```python
from build123d import *

# Parameters (mm, degrees)
BOSS_EXTRUDE1_DEPTH = 10
SKETCH4_R           = 2
CUT_EXTRUDE2_DEPTH  = 10


with BuildPart() as part:
    # Sketch1 → Boss-Extrude1 (new body)
    with BuildSketch(Plane.XY):
        Polygon((33.476154754, 62), (-33.476154754, 62), (-33.5, 62), (-33.5, 3), (-48.5, 3), (-48.5, 0), (-28.5, 0), (-28.5, 57), (28.5, 57), (28.5, 0), (48.5, 0), (48.5, 3), (33.5, 3), (33.5, 62), align=None)
    extrude(amount=BOSS_EXTRUDE1_DEPTH)

    # Sketch4 → Cut-Extrude2 (cut)
    with BuildSketch(Plane(origin=(0, 0, 0), x_dir=(1, 0, 0), z_dir=(0, 1, 0))):
        with Locations((-41.522360656, -5)):
            Circle(SKETCH4_R)
        with Locations((41.522360656, -5)):
            Circle(SKETCH4_R)
    extrude(amount=CUT_EXTRUDE2_DEPTH, mode=Mode.SUBTRACT)


solid = part.part
```
Input: part model. Units: mm. Frame: model coordinates. A direction names the side the tool comes from. Give positions to 0.01 mm unless a question says otherwise; leave off trailing zeros. Loops run counter-clockwise (first coordinate to the right, second up) from the corner with the lowest first, then second, coordinate; pieces in that order, holes last. Notation, with made-up numbers: (58, 44) -> (90, 44) arc R18 ccw to (90, 77) -> close; hole circle Ø7 at (-30, 89). An arc over 180 degrees is marked (long way). Use a Markdown table: item, result.
Q1. Section query B-B, the plane z = 5. Return the cut outline in (x, y).
Entries:
| item | result |
|---|---|
| outline | (-48.5, 0) -> (-43.52, 0) -> (-43.52, 3) -> (-48.5, 3) -> close; (-39.52, 0) -> (-28.5, 0) -> (-28.5, 57) -> (28.5, 57) -> (28.5, 0) -> (39.52, 0) -> (39.52, 3) -> (33.5, 3) -> (33.5, 62) -> (-33.5, 62) -> (-33.5, 3) -> (-39.52, 3) -> close; (43.52, 0) -> (48.5, 0) -> (48.5, 3) -> (43.52, 3) -> close |
Q2. Section query C-C, the plane x = 22.5. Return the cut outline in (y, z), plus the area to 3 significant figures.
Entries:
| item | result |
|---|---|
| outline | (57, 0) -> (62, 0) -> (62, 10) -> (57, 10) -> close |
| area | 50.0 mm² |
Q3. Access query for faces 4 (the flat face through (28.5, 29, 5)), 5 (the flat face through (-33.5, 33, 5)), 6 (the flat face through (38, 0, 5)). Directions: +Z, -Z, +X, -X, +Y, -Y. A direction counts if a zero-diameter tool reaches every point of the face in a straight line with its end or side. Return the directions, or none.
Entries:
| item | result |
|---|---|
| face 4 | +Z, -Z, -Y |
| face 5 | +Z, -Z, -X, +Y |
| face 6 | +Z, -Z, +X, -X, -Y |
Q4. Ray query, probe 1 along X at (y, z) = (2, 5); probe 2 along X at (y, z) = (45.5, 3.25); probe 3 along Y at (x, z) = (-1, 8.75). Return the intervals inside material, ascending. Write a range as from..to.
Entries:
| item | result |
|---|---|
| probe 1 | x = -48.5..-43.52, -39.52..-28.5, 28.5..39.52, 43.52..48.5 |
| probe 2 | x = -33.5..-28.5, 28.5..33.5 |
| probe 3 | y = 57..62 |
Q5. First-contact query: P1, Ø5, axis at y = 34.5, z = 5.5, coming from the +X side; P2, Ø3, axis at x = 41.52, z = 5, coming from the +Y side; P3, Ø5, axis at x = 44.5, z = 4, coming from the +Y side. Flat tips, straight axial feed; report the tip coordinate or a pass-through.
Entries:
| item | result |
|---|---|
| P1 | stops at x = 33.5 |
| P2 | passes through |
| P3 | stops at y = 3 |
Q6. Section query D-D, the plane y = 58.5. Return the cut outline in (x, z), plus the area to 3 significant figures.
Entries:
| item | result |
|---|---|
| outline | (-33.5, 0) -> (33.5, 0) -> (33.5, 10) -> (-33.5, 10) -> close |
| area | 670 mm² |
Q7. Section query A-A, the plane y = 37.5. Return the cut outline in (x, z), plus the area to 3 significant figures.
Entries:
| item | result |
|---|---|
| outline | (-33.5, 0) -> (-28.5, 0) -> (-28.5, 10) -> (-33.5, 10) -> close; (28.5, 0) -> (33.5, 0) -> (33.5, 10) -> (28.5, 10) -> close |
| area | 100 mm² |
Q8. Pull-direction query (X, two-part tool) for faces 1 (the flat face through (-28.5, 28, 5)), 2 (the flat face through (39, 3, 5)), 3 (the flat face through (33.5, 32, 5)); classes: pulls with the +X half, pulls with the -X half, needs draft (parallel to the pull), parting line crosses it, or undercut.
Entries:
| item | result |
|---|---|
| face 1 | undercut |
| face 2 | needs draft |
| face 3 | pulls with the +X half |
